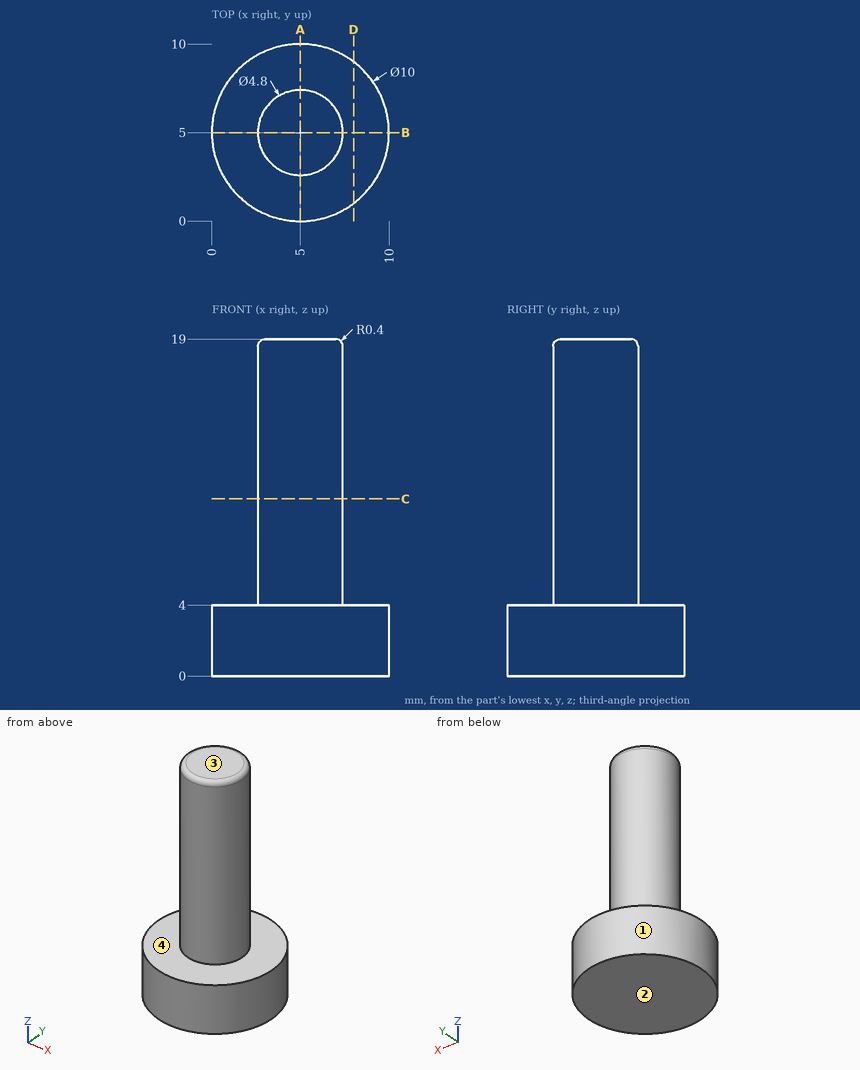
The figure shows three views and two pictorial views of one solid part (mm, origin at its lowest corner). Answer the questions. A direction names the side the tool comes from. Give positions to 0.01 mm unless a question says otherwise; leave off trailing zeros. Order: outer loops, then holes, each group sorted by start corner. A loop starts at its lowest first (then second) coordinate and runs counter-clockwise, first axis right, second up. Notation, with made-up numbers: (-32, -5) -> (-12, -5) arc R6 cw to (-12, 1) -> close; hole circle Ø5 at (28, 87). An arc over 180 degrees is marked (long way). One line per item, written item: value.
1) Find section C-C, the plane z = 10. Determine the outline of the cut face in (x, y), plus the area to 3 significant figures.
Reported:
outline: circle Ø4.8 at (5, 5)
area: 18.1 mm^2
2) Find section A-A, the plane x = 5. Determine the outline of the cut face in (y, z), plus the area to 3 significant figures.
Reported:
outline: (0, 0) -> (10, 0) -> (10, 4) -> (7.4, 4) -> (7.4, 18.6) arc R0.4 ccw to (7, 19) -> (3, 19) arc R0.4 ccw to (2.6, 18.6) -> (2.6, 4) -> (0, 4) -> close
area: 112 mm^2
3) Find section D-D, the plane x = 8. Determine the outline of the cut face in (y, z), plus the area to 3 significant figures.
Reported:
outline: (1, 0) -> (9, 0) -> (9, 4) -> (1, 4) -> close
area: 32.0 mm^2
4) Determine the mould class of the marked faces 1 and 2 for opening direction X: pulls with the +X half, pulls with the -X half, needs draft (parallel to the pull), parting line crosses it, or undercut.
Reported:
face 1: parting line crosses it
face 2: needs draft
5) Find the intervals of material crossed by line 1 (Z direction, x = 4.75, y = 9.25); line 2 (Y direction, x = 5, z = 5); line 3 (X direction, y = 7.75, z = 2.75), in increasing order.
Reported:
line 1: z = 0 to 4
line 2: y = 2.6 to 7.4
line 3: x = 0.82 to 9.18
6) Flat-ended cylindrical pins translate along their axes: P1, Ø1, axis at x = 4, z = 10.5, coming from the +Y side; P2, Ø2, axis at y = 3, z = 13.5, coming from the +X side; P3, Ø3, axis at x = 8, y = 5.5, coming from the -Z side; P4, Ø3, axis at y = 5.5, z = 6, coming from the -X side. Find the tip coordinate at first contact, or state that the pin passes through.
Reported:
P1: stops at y = 7.35
P2: stops at x = 7.18
P3: stops at z = 0
P4: stops at x = 2.6
7) A tool of negligible diameter and unlimited length cuts with its end or side. For the marked faces 3 and 4, from which of +Z, -Z, +X, -X, +Y, -Y can it reach the whole face along a straight path? Write none if from no direction.
Reported:
face 3: +Z, +X, -X, +Y, -Y
face 4: +Z
